```python
from build123d import *

# Parameters (mm, degrees)
F1_DEPTH  = 10
F2_W      = 110
F2_H      = 10
F3_DEPTH  = 50
F4_W      = 10
F4_H      = 44
F5_DEPTH  = 50
F7_DEPTH  = 11
F9_DEPTH  = 25
F10_R     = 6
F11_DEPTH = 11
F13_DEPTH = 11


with BuildPart() as f1:
    # F0 (on Front) → F1 (new body)
    with BuildSketch(Plane.XZ):
        Polygon((35.2384935319, 27.3238807813), (-74.7615064681, 27.3238807813), (-74.7615064681, 7.3238807813), (-22.7615064681, -26.6761192187), (35.2384935319, -26.6761192187), align=None)
    extrude(amount=F1_DEPTH)

    # F2 (on face) → F3 (join)
    with BuildSketch(Plane.XZ.offset(10)):
        with Locations((-19.7615064681, 22.3238807813)):
            Rectangle(F2_W, F2_H)
    extrude(amount=F3_DEPTH)

    # F4 (on face) → F5 (join)
    with BuildSketch(Plane.XZ.offset(10)):
        with Locations((-17.7615064681, -4.6761192187)):
            Rectangle(F4_W, F4_H)
    extrude(amount=F5_DEPTH)

    # F6 (on face) → F7 (cut)
    with BuildSketch(Plane.YZ.offset(-12.7615064681)):
        Polygon((-10, -26.6761192187), (-60, 17.3238807813), (-60, -26.6761192187), align=None)
    extrude(amount=-F7_DEPTH, mode=Mode.SUBTRACT)

    # F8 (on face) → F9 (cut)
    with BuildSketch(Plane(origin=(0, 0, 17.3238807813), x_dir=(1, 0, 0), z_dir=(0, 0, -1))):
        Polygon((35.2384935319, 60), (-12.7615064681, 60), (35.2384935319, 10), align=None)
    extrude(amount=-F9_DEPTH, mode=Mode.SUBTRACT)

    # F10 (on face) → F11 (cut)
    with BuildSketch(Plane.XZ.offset(10)):
        with Locations((23.2384935319, -4.6761192187)):
            Circle(F10_R)
        with Locations((1.2384935319, -4.6761192187)):
            Circle(F10_R)
    extrude(amount=-F11_DEPTH, mode=Mode.SUBTRACT)

    # F12 (on face) → F13 (cut)
    with BuildSketch(Plane(origin=(0, 0, 17.3238807813), x_dir=(1, 0, 0), z_dir=(0, 0, -1))):
        with BuildLine():
            ThreePointArc((-53.7615064681, 46), (-58.7615064681, 51), (-63.7615064681, 46))
            Line((-63.7615064681, 46), (-63.7615064681, 26))
            ThreePointArc((-63.7615064681, 26), (-58.7615064681, 21), (-53.7615064681, 26))
            Line((-53.7615064681, 26), (-53.7615064681, 46))
        make_face()
        with BuildLine():
            Line((-41.7615064681, 46), (-41.7615064681, 26))
            ThreePointArc((-41.7615064681, 26), (-36.7615064681, 21), (-31.7615064681, 26))
            Line((-31.7615064681, 26), (-31.7615064681, 46))
            ThreePointArc((-31.7615064681, 46), (-36.7615064681, 51), (-41.7615064681, 46))
        make_face()
    extrude(amount=-F13_DEPTH, mode=Mode.SUBTRACT)


solid = f1.part
```
Work out the finished part from the listing and answer in its coordinate system (mm). A direction names the side the tool comes from. Give positions to 0.01 mm unless a question says otherwise; leave off trailing zeros. Order: outer loops, then holes, each group sorted by start corner. A loop starts at its lowest first (then second) coordinate and runs counter-clockwise, first axis right, second up. Notation, with made-up numbers: (10, -30.5) -> (63, -30.5) arc R29 ccw to (63, 7.5) -> close; hole circle Ø1 at (-14.5, 14.5). An arc over 180 degrees is marked (long way). Answer as CSV lines item,"result". Start each with the question number.
(1) Consider line 1 along X through (y, z) = (-24.5, 24); line 2 along Y through (x, z) = (-0.5, 9); line 3 along X through (y, z) = (-2.5, -4.5). Determine where each line is inside the solid, lowest interval first.
(2) Each of these flat-tipped pins is pushed along its axis until it touches: pin 1 Ø3 at (y, z) = (-33.5, 20) entering from +X; pin 2 Ø22 at (y, z) = (-46.5, 2) entering from -X; pin 3 Ø19 at (x, z) = (1.24, -4.68) entering from -Y. Where does it stop, or does it pass through?
(3) Section B-B, the plane y = -6 is taken. Write down the section's boundary in (x, z), plus the area to 3 significant figures.
(4) Which of the six approach directions +Z, -Z, +X, -X, +Y, -Y give full straight-line access (tool end or side, diameter ignored) to faces 5 (the flat face through (-17.692, -34.65, -4.984)), 6 (the flat face through (-43, -10, 1)), 7 (the flat face through (-21, -23, 27.324)), 8 (the flat face through (-63.762, -36, 22)), 9 (the flat face through (6, -29, 17.324))?
(5) Section D-D, the plane x = -14 is taken. Write down the section's boundary in (y, z).
(6) Section C-C, the plane z = -2 is taken. Write down the section's boundary in (x, y), plus the area to 3 significant figures.
(7) Section A-A, the plane x = -62 is taken. Write down the section's boundary in (y, z), plus the area to 3 significant figures.
(8) For a pull along X with two mould halves and no side action, classify faces 1 (the flat face through (-22.762, -24, 5)), 2 (the flat face through (-49, -35, 17.324)), 3 (the flat face through (-12.762, -24, 5)), 4 (the flat face through (-53.762, -36, 22)) as released by +X, released by -X, zero draft, split by the parting line, or undercut.
Entries:
1,line 1,"-74.76 to -63.53, -53.99 to -41.53, -31.99 to 21.32"
1,line 2,"-10 to 0"
1,line 3,"-56.68 to -4.76, 7.24 to 17.24, 29.24 to 35.24"
2,pin 1,"x = 14.12"
2,pin 2,"x = -22.76"
2,pin 3,"y = -10"
3,outline,"(-74.76, 7.32) -> (-22.76, -26.68) -> (35.24, -26.68) -> (35.24, 27.32) -> (-74.76, 27.32) -> close; hole circle Ø12 at (1.24, -4.68); hole circle Ø12 at (23.24, -4.68)"
3,area,"4,830 mm²"
4,face 5,"-Z, +X, -X, -Y"
4,face 6,"-Z, -X, -Y"
4,face 7,"+Z, +X, -X, +Y, -Y"
4,face 8,"+Z, -Z"
4,face 9,"-Z, +X, -Y"
5,outline,"(-60, 17.32) -> (-10, -26.68) -> (0, -26.68) -> (0, 27.32) -> (-60, 27.32) -> close"
6,outline,"(-60.5, -10) -> (-22.76, -10) -> (-22.76, -38.04) -> (-12.76, -38.04) -> (-12.76, -10) -> (-4.13, -10) -> (-4.13, 0) -> (-60.5, 0) -> close; (6.61, -10) -> (17.87, -10) -> (17.87, 0) -> (6.61, 0) -> close; (28.61, -10) -> (35.24, -10) -> (35.24, 0) -> (28.61, 0) -> close"
6,area,"1,020 mm²"
7,outline,"(-60, 17.32) -> (-49.81, 17.32) -> (-49.81, 27.32) -> (-60, 27.32) -> close; (-22.19, 17.32) -> (-10, 17.32) -> (-10, -1.02) -> (0, -1.02) -> (0, 27.32) -> (-22.19, 27.32) -> close"
7,area,"507 mm²"
8,face 1,"released by -X"
8,face 2,"zero draft"
8,face 3,"released by +X"
8,face 4,"undercut"
